```python
from build123d import *

# Parameters (mm, degrees)
SKETCH1_R                = 21.5
SKETCH1_R_2              = 14
BOSS_EXTRUDE1_DEPTH      = 4
BOSS_EXTRUDE2_REACH      = 50.242
BOSS_EXTRUDE2_END_RADIUS = 21.5
SKETCH2_W                = 4
SKETCH2_H                = 43
SKETCH2_3_W              = 45
SKETCH2_3_H              = 43
SKETCH2_3_R              = 3
BOSS_EXTRUDE3_DEPTH      = 5
CUT_EXTRUDE4_DEPTH       = 64.184254368
WIRE_BREAK_DEPTH         = 54.343228249


with BuildPart() as part:
    # Sketch1 → Boss-Extrude1 (new body)
    with BuildSketch(Plane(origin=(0, 0, 0), x_dir=(0, 0, -1), z_dir=(1, 0, 0))):
        Circle(SKETCH1_R)
        Circle(SKETCH1_R_2, mode=Mode.SUBTRACT)
    extrude(amount=BOSS_EXTRUDE1_DEPTH)

    # Boss-Extrude2: up to this cylinder (the profile starts outside it)
    boss_extrude2_end = Plane(origin=(2, 0, 0), z_dir=(-1, 0, 0)) * Cylinder(BOSS_EXTRUDE2_END_RADIUS, 144.484, mode=Mode.PRIVATE)
    # Sketch2 → Boss-Extrude2 (add, up to the surface)
    with BuildSketch(Plane(origin=(0, 21.5, 0), x_dir=(1, 0, 0), z_dir=(0, 1, 0)), mode=Mode.PRIVATE) as boss_extrude2_sk1:
        with Locations((2, 0)):
            Rectangle(SKETCH2_W, SKETCH2_H)
    boss_extrude2_tool1 = extrude(boss_extrude2_sk1.sketch, amount=-BOSS_EXTRUDE2_REACH, mode=Mode.PRIVATE) - boss_extrude2_end
    add(boss_extrude2_tool1.solids().sort_by_distance((2, 21.5, 0))[0])
    add(boss_extrude2_tool1.solids().sort_by_distance((2, 21.5, 0))[1])

    # Sketch2_3 → Boss-Extrude3 (add)
    with BuildSketch(Plane(origin=(0, 21.5, 0), x_dir=(1, 0, 0), z_dir=(0, 1, 0))):
        with Locations((-18.5, 0)):
            Rectangle(SKETCH2_3_W, SKETCH2_3_H)
        with Locations(Location((-36, 0, 0), (0, 0, 270))):
            Circle(SKETCH2_3_R, mode=Mode.SUBTRACT)
    extrude(amount=BOSS_EXTRUDE3_DEPTH)

    # Sketch3 → Cut-Extrude4 (cut, through all)
    with BuildSketch(Plane.XZ.offset(-21.5)):
        Polygon((0, -28.471778575), (0, -21.5), (-41, -7.216009452), (-41, -28.471778575), align=None)
        Polygon((-41, 7.216009452), (0, 21.5), (0, 27.25128432), (-41, 27.25128432), align=None)
    extrude(amount=-CUT_EXTRUDE4_DEPTH, mode=Mode.SUBTRACT)

    # Sketch4 → wire break (cut, through all)
    with BuildSketch(Plane.ZY):
        Polygon((-3.959672524, 3.053030216), (3.959672524, -3.053030216), (-14.358508771, -26.811065363), (-22.27785382, -20.705004931), align=None)
    extrude(amount=-WIRE_BREAK_DEPTH, mode=Mode.SUBTRACT)


solid = part.part
```
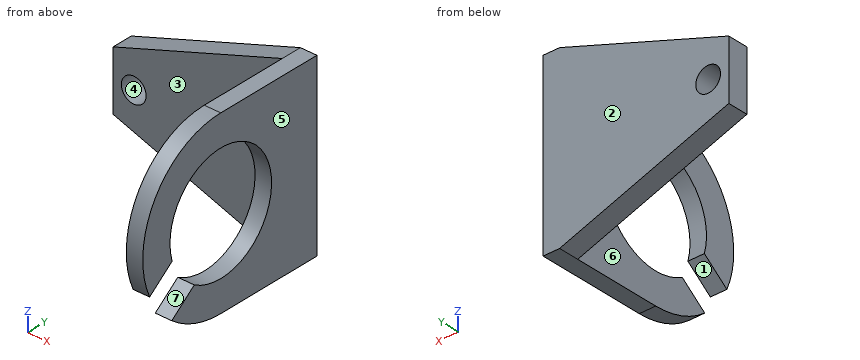
Here's how the part is built. I have some questions about the finished solid (model axes, mm). Face numbers are marked on the shaded views. A direction names the side the tool comes from. Coordinates: 2 decimals unless noted, no trailing zeros. Order: outer loops, then holes, each group sorted by start corner. A loop starts at its lowest first (then second) coordinate and runs counter-clockwise, first axis right, second up.
1) Imagine slicing it at C-C on y = -12. List the corners of the cut face in (x, z) for me.
2) Which directions (+Z, -Z, +X, -X, +Y, -Y) give clear straight access to the entire face, cutting with the end or side of a thin tool? Please do the marked faces 5, 6 and 7.
3) I need wall thicknesses on line 1 (Y direction, x = 1.65, z = 0); line 2 (X direction, y = 24, z = 0); line 3 (Y direction, x = -4, z = 8.5). Which ranges of each line are inside material? Lowest first, please.
4) Imagine slicing it at D-D on y = 17. List the corners of the cut face in (x, z) for me.
5) Imagine slicing it at A-A on z = 0. List the corners of the cut face in (x, y) for me, and give its area (3 significant figures).
6) We'd pull the mould along Y, two halves only. Please class the marked faces 1, 2, 3 and 4: +Y half, -Y half, draft (parallel to the pull), parting line (faces both ways), or undercut.
7) Will these pins go through, and if not, where does the flat tip stop? pin 1 (4 mm diameter, centred on y = -11, z = 8.5, fed in from -X); pin 2 (10 mm diameter, centred on y = 8.5, z = 5.5, fed in from +X); pin 3 (5 mm diameter, centred on x = -23.5, z = 11.5, fed in from -Y); pin 4 (5 mm diameter, centred on x = -36, z = 0, fed in from -Y).
8) Imagine slicing it at B-B on x = -36. List the corners of the cut face in (y, z) for me.
Response values:
1. outline: (0, -17.84) - (4, -17.84) - (4, -15.57) - (0, -15.57) - close; (0, 7.21) - (4, 7.21) - (4, 17.84) - (0, 17.84) - close
2. face 5: +Z, -Z, +X, +Y, -Y
2. face 6: +Z, -Z, -X, -Y
2. face 7: +X, -X, -Y
3. line 1: y = -21.5 to -14, 14 to 26.5
3. line 2: x = -41 to -39, -33 to 4
3. line 3: y = 21.5 to 26.5
4. outline: (0, -21.5) - (4, -21.5) - (4, 21.5) - (0, 21.5) - close
5. outline: (-41, 21.5) - (-39, 21.5) - (-39, 26.5) - (-41, 26.5) - close; (-33, 21.5) - (0, 21.5) - (0, 14) - (4, 14) - (4, 26.5) - (-33, 26.5) - close; (0, -21.5) - (4, -21.5) - (4, -14) - (0, -14) - close
5. area: 255 mm2
6. face 1: undercut
6. face 2: +Y half
6. face 3: -Y half
6. face 4: draft
7. pin 1: stops at x = 0
7. pin 2: stops at x = 4
7. pin 3: stops at y = 21.5
7. pin 4: passes through
8. outline: (21.5, -8.96) - (26.5, -8.96) - (26.5, -3) - (21.5, -3) - close; (21.5, 3) - (26.5, 3) - (26.5, 8.96) - (21.5, 8.96) - close
